For this review, take the finished solid that the model builds, in its own axes (mm). A direction names the side the tool comes from. Round coordinates to 2 decimals unless told otherwise and drop trailing zeros. Loops run counter-clockwise (first coordinate to the right, second up) from the corner with the lowest first, then second, coordinate; pieces in that order, holes last. Notation, with made-up numbers: (18.5, 13) -> (61.5, 13) arc R22 ccw to (61.5, 50) -> close; hole circle Ø6 at (-27.5, 72). An arc over 180 degrees is marked (long way). Write each question's results on one line, items separated by ' | '.
```python
from build123d import *

# Parameters (mm, degrees)
F0_W     = 90
F0_H     = 90
F1_DEPTH = 13
F3_DEPTH = 25
F4_D     = 8.8
F4_DEPTH = 18.25
F4_TIP   = 2.6437867237


with BuildPart() as f1:
    # F0 (on Front) → F1 (new body)
    with BuildSketch(Plane.XZ):
        with Locations((45, -45)):
            Rectangle(F0_W, F0_H)
    extrude(amount=F1_DEPTH)

    # F2 (on face) → F3 (cut)
    with BuildSketch(Plane.XZ.offset(13)):
        with BuildLine():
            Line((71.4366715828, -59.2910452421), (71.4366715828, -60.7089547579))
            ThreePointArc((71.4366715828, -60.7089547579), (71.5, -60), (71.4366715828, -59.2910452421))
        make_face()
        with BuildLine():
            Line((71.4366715828, -74.2910452421), (71.4366715828, -60.7089547579))
            Line((71.4366715828, -60.7089547579), (71.4366715828, -59.2910452421))
            ThreePointArc((71.4366715828, -59.2910452421), (67.1441112051, -56.0158635609), (63.5, -60))
            Line((63.5, -60), (63.5, -75))
            ThreePointArc((63.5, -75), (67.8558887949, -78.9841364391), (71.4366715828, -74.2910452421))
        make_face()
        with BuildLine():
            Line((26.5, -75), (26.5, -60))
            ThreePointArc((26.5, -60), (22.4956317773, -56.0000023852), (18.5000095407, -60.0087364402))
            Line((18.5000095407, -60.0087364402), (18.5316552492, -74.4977650565))
            ThreePointArc((18.5316552492, -74.4977650565), (22.2483842248, -78.9920783436), (26.5, -75))
        make_face()
    extrude(amount=-F3_DEPTH, mode=Mode.SUBTRACT)

    # F4
    with Locations(Plane.XZ.offset(13)):
        with Locations((22.5, -22.5), (67.5, -22.5)):
            Hole(F4_D / 2, depth=F4_DEPTH)
            with Locations((0, 0, -(F4_DEPTH + F4_TIP / 2))):  # 118° drill point
                Cone(0, F4_D / 2, F4_TIP, mode=Mode.SUBTRACT)


solid = f1.part
```
1. Consider section C-C (y = -9.5). State the section outline as (x, z) points, plus the area to 3 significant figures.
Values found:
outline: (0, -90) -> (90, -90) -> (90, 0) -> (0, 0) -> close; hole circle Ø8.8 at (22.5, -22.5); hole (18.5, -60.01) -> (18.53, -74.5) arc R4 ccw (long way) to (26.5, -75) -> (26.5, -60) arc R4 ccw to start; hole circle Ø8.8 at (67.5, -22.5); hole (63.5, -75) arc R4 ccw (long way) to (71.44, -74.29) -> (71.44, -60.71) arc R4 ccw (long way) to (63.5, -60) -> close | area: 7,640 mm2
2. Consider section A-A (x = 22.5). State the section outline as (y, z) points.
Values found:
outline: (-13, -90) -> (0, -90) -> (0, -79) -> (-13, -79) -> close; (-13, -56) -> (0, -56) -> (0, -26.9) -> (-13, -26.9) -> close; (-13, -18.1) -> (0, -18.1) -> (0, 0) -> (-13, 0) -> close
3. To check wall thickness, follow probe 1 along X at (y, z) = (-6, -63); probe 2 along Z at (x, y) = (67.5, -5.25); probe 3 along Z at (x, y) = (24, -9.5). State the ranges of each line that lie inside material, in increasing order.
Values found:
probe 1: x = 0 to 18.51, 26.5 to 63.5, 71.44 to 90 | probe 2: z = -90 to -79, -56 to -26.9, -18.1 to 0 | probe 3: z = -90 to -78.71, -56.29 to -26.64, -18.36 to 0
4. Tool access review of faces 1 (the face through (26.5, -7, -68)), 2 (the face through (0, -6, -46)): name each direction out of +Z, -Z, +X, -X, +Y, -Y from which nothing blocks a thin tool from reaching the whole face with its end or side.
Values found:
face 1: +Y, -Y | face 2: +Z, -Z, -X, +Y, -Y
5. Draft analysis for pull direction Z (two halves, no side actions). For faces 3 (the face through (22.6, -6.6, -56)), 4 (the face through (44, -6, -90)), 5 (the face through (63.5, -7, -67)), 6 (the face through (44, 0, -44)), state which applies: released by +Z, released by -Z, zero draft, split by the parting line, or undercut.
Values found:
face 3: undercut | face 4: released by -Z | face 5: undercut | face 6: zero draft
6. Consider section B-B (z = -22.5). State the section outline as (x, y) points, plus the area to 3 significant figures.
Values found:
outline: (0, -13) -> (18.1, -13) -> (18.1, 0) -> (0, 0) -> close; (26.9, -13) -> (63.1, -13) -> (63.1, 0) -> (26.9, 0) -> close; (71.9, -13) -> (90, -13) -> (90, 0) -> (71.9, 0) -> close | area: 941 mm2
7. For pin 1 (7 mm diameter, centred on x = 67.5, z = -75, fed in from -Y), flat-tipped, find the tip position at first contact; note if it passes through.
Values found:
pin 1: passes through
